Work out the finished part from the listing and answer in its coordinate system (mm). A direction names the side the tool comes from. Give positions to 0.01 mm unless a question says otherwise; leave off trailing zeros. Loops run counter-clockwise (first coordinate to the right, second up) from the corner with the lowest first, then second, coordinate; pieces in that order, holes last. Notation, with made-up numbers: (79, 41.25) - (88, 41.25) arc R23 ccw to (88, 62.25) - close; hole circle Ø1 at (54.5, 76). An arc over 180 degrees is marked (long way). Use CSV: the item, a comma, the result in double quotes.
from build123d import *

# Parameters (mm, degrees)
F1_DEPTH = 30.1625
F2_R     = 1.5875
F3_DEPTH = 25.4
F4_R     = 1.5875
F4_R_2   = 10.31875
F5_DEPTH = 25.4


with BuildPart() as f1:
    # F0 (on Top) → F1 (new body)
    with BuildSketch(Plane.XY):
        Polygon((17.641182, 19.748247), (-28.396318, 19.748247), (-28.396318, 16.573247), (17.641182, 16.573247), (17.641182, 15.779497), (49.391182, 15.779497), (49.391182, 20.541997), (17.641182, 20.541997), align=None)
    extrude(amount=F1_DEPTH)

    # F2 (on face) → F3 (cut)
    with BuildSketch(Plane.XZ.offset(-16.573247)):
        with Locations((-25.221318, 15.08125)):
            Circle(F2_R)
        with BuildLine():
            ThreePointArc((-28.396318, 15.08125), (-26.367545, 18.042127), (-22.873931, 17.219099))
            ThreePointArc((-22.873931, 17.219099), (-22.312971, 16.823539), (-21.63746, 16.701765))
            Line((-21.63746, 16.701765), (13.280901, 18.083688))
            ThreePointArc((13.280901, 18.083688), (15.992776, 19.064871), (17.641182, 21.43125))
            Line((17.641182, 21.43125), (17.641182, 30.1625))
            Line((17.641182, 30.1625), (-28.396318, 30.1625))
            Line((-28.396318, 30.1625), (-28.396318, 15.08125))
        make_face()
        with BuildLine():
            ThreePointArc((-21.63746, 13.460735), (-22.312971, 13.338961), (-22.873931, 12.943401))
            ThreePointArc((-22.873931, 12.943401), (-26.367545, 12.120373), (-28.396318, 15.08125))
            Line((-28.396318, 15.08125), (-28.396318, 0))
            Line((-28.396318, 0), (17.641182, 0))
            Line((17.641182, 0), (17.641182, 8.73125))
            ThreePointArc((17.641182, 8.73125), (15.992776, 11.097629), (13.280901, 12.078812))
            Line((13.280901, 12.078812), (-21.63746, 13.460735))
        make_face()
    extrude(amount=-F3_DEPTH, mode=Mode.SUBTRACT)

    # F4 (on face) → F5 (cut)
    with BuildSketch(Plane.XZ.offset(-15.779497)):
        with Locations((-25.221318, 15.08125)):
            Circle(F4_R)
        with BuildLine():
            ThreePointArc((44.311182, 25.24125), (48.050407, 20.760863), (49.391182, 15.08125))
            Line((49.391182, 15.08125), (49.391182, 30.1625))
            Line((49.391182, 30.1625), (43.041182, 30.1625))
            Line((43.041182, 30.1625), (43.041182, 27.78125))
            ThreePointArc((43.041182, 27.78125), (43.376375, 26.361347), (44.311182, 25.24125))
        make_face()
        Polygon((30.341182, 27.78125), (30.341182, 30.1625), (17.641182, 30.1625), (17.641182, 21.43125), (23.991182, 21.43125), (23.991182, 27.78125), align=None)
        with BuildLine():
            Line((49.391182, 0), (49.391182, 15.08125))
            ThreePointArc((49.391182, 15.08125), (48.050407, 9.401637), (44.311182, 4.92125))
            ThreePointArc((44.311182, 4.92125), (43.376375, 3.801153), (43.041182, 2.38125))
            Line((43.041182, 2.38125), (43.041182, 0))
            Line((43.041182, 0), (49.391182, 0))
        make_face()
        with BuildLine():
            Line((17.641182, 0), (30.341182, 0))
            Line((30.341182, 0), (30.341182, 2.38125))
            ThreePointArc((30.341182, 2.38125), (30.005988, 3.801153), (29.071182, 4.92125))
            ThreePointArc((29.071182, 4.92125), (27.710925, 6.100994), (26.531182, 7.46125))
            ThreePointArc((26.531182, 7.46125), (25.411085, 8.396056), (23.991182, 8.73125))
            Line((23.991182, 8.73125), (17.641182, 8.73125))
            Line((17.641182, 8.73125), (17.641182, 0))
        make_face()
        with Locations((36.691182, 15.08125)):
            Circle(F4_R_2)
    extrude(amount=-F5_DEPTH, mode=Mode.SUBTRACT)


solid = f1.part
Item 1: The mould has two halves that part along Z. Classify faces 4 (the cylindrical face through (26.382, 18.127, 15.535)), 5 (the cylindrical face through (-23.755, 18.139, 14.473)), 6 (the cylindrical face through (43.386, 18.127, 3.82)), 7 (the cylindrical face through (43.367, 18.127, 26.38)): pulls with the +Z half, pulls with the -Z half, needs draft (parallel to the pull), parting line crosses it, or undercut.
Determined:
face 4,"undercut"
face 5,"undercut"
face 6,"pulls with the -Z half"
face 7,"pulls with the +Z half"
Item 2: For faces 1 (the flat face through (43.041, 18, 29)), 2 (the flat face through (-2, 19.748, 15)), 3 (the flat face through (30.341, 18, 29)), determine the directions among +Z, -Z, +X, -X, +Y, -Y from which every point of the face is accessible in a straight line to the end or side of a thin tool.
Determined:
face 1,"+Z, +X, +Y, -Y"
face 2,"+Z, -Z, -X, +Y"
face 3,"+Z, -X, +Y, -Y"
Item 3: A cutting plane is placed at C-C on x = 21. Determine the outline of the cut face in (y, z), and give its area (3 significant figures).
Determined:
outline,"(15.78, 8.73) - (20.54, 8.73) - (20.54, 21.43) - (15.78, 21.43) - close"
area,"60.5 mm²"
Item 4: A cutting plane is placed at A-A on y = 17.4. State how many separate pieces and enclosed holes the cut face has, and give its area (3 significant figures).
Determined:
separate pieces,"1"
enclosed holes,"2"
area,"585 mm²"
Item 5: Given P1, Ø2.5, axis at y = 17.5, z = 29.5, coming from the -X side; P2, Ø10, axis at x = -13.5, z = 17, coming from the -Y side; P3, Ø14, axis at x = -10, z = 14, coming from the +Y side; P4, Ø0.6, axis at y = 16.5, z = 15, coming from the -X side, each flat-ended and moving along its own axis, determine where each tip first touches the part or whether it passes through.
Determined:
P1,"stops at x = 30.34"
P2,"stops at y = 16.57"
P3,"stops at y = 19.75"
P4,"stops at x = -28.4"
Item 6: A cutting plane is placed at B-B on z = 6.5. Determine the outline of the cut face in (x, y).
Determined:
outline,"(27.33, 15.78) - (30.96, 15.78) - (30.96, 20.54) - (27.33, 20.54) - close; (42.42, 15.78) - (46.05, 15.78) - (46.05, 20.54) - (42.42, 20.54) - close"
Item 7: A cutting plane is placed at D-D on z = 20.5. Determine the outline of the cut face in (x, y).
Determined:
outline,"(17.24, 16.57) - (17.64, 16.57) - (17.64, 15.78) - (27.91, 15.78) - (27.91, 20.54) - (17.64, 20.54) - (17.64, 19.75) - (17.24, 19.75) - close; (45.47, 15.78) - (48.18, 15.78) - (48.18, 20.54) - (45.47, 20.54) - close"
Item 8: Find the intervals of material crossed by line 1 (X direction, y = 19.15, z = 14.5); line 2 (Z direction, x = 38.5, y = 18.5); line 3 (X direction, y = 16.5, z = 19.5), in increasing order.
Determined:
line 1,"x = -28.34 to -26.7, -23.74 to 26.39, 46.99 to 49.38"
line 2,"z = 0 to 4.92, 25.24 to 30.16"
line 3,"x = 17.64 to 27.37, 46.02 to 48.6"
